Build history of the part. All positions in model axes, mm. Give positions to 0.01 mm unless a question says otherwise; leave off trailing zeros. Write each loop counter-clockwise with the first axis right and the second up, starting at its lowest first coordinate (ties: lowest second). Pieces come first, ordered by that corner, then holes. Notation, with made-up numbers: (-5.75, 49) -> (6.25, 49) arc R22 ccw to (6.25, 88) -> close; hole circle Ø3 at (16, 14). An arc over 180 degrees is marked (long way). One line per question, with ' | ' between items. Start each with the question number.
(1) Band-saw the part on A-A, the plane x = 168.5. Give the cut face in (y, z), and give its area (3 significant figures).
(2) Drill centre lines: probe 1 along X at (y, z) = (162, 5) (3 decimals); probe 2 along Y at (x, z) = (19.05, 2.5); probe 3 along Y at (x, z) = (69, 5.75). Where is each one in solid material? Low to high. Write a range as from..to.
(3) Pin check, flat tips, straight feed: P1, Ø7.5, axis at x = 19.05, y = 127, coming from the +Z side; P2, Ø3, axis at x = 65.5, z = 3, coming from the -Y side; P3, Ø2, axis at y = 90, z = 2, coming from the -X side. Stop position of each tip, or through.
(4) Band-saw the part on C-C, the plane x = 49. Give the cut face in (y, z), and give its area (3 significant figures).
(5) Band-saw the part on B-B, the plane z = 2.5. Count the separate pieces of the cut face and the enclosed holes in it, and give its area (3 significant figures).
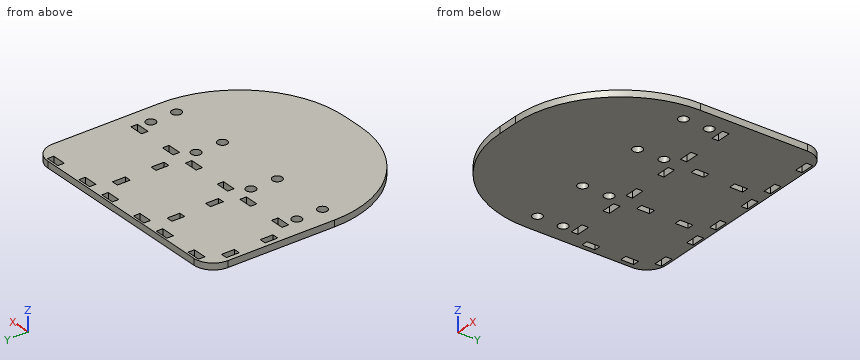
from build123d import *

# Parameters (mm, degrees)
SKETCH1_W               = 228.6
SKETCH1_H               = 228.6
BOSS_EXTRUDE1_DEPTH     = 6.35
CUT_EXTRUDE1_DEPTH      = 324.351577234
CUT_EXTRUDE1_DEPTH_BACK = 324.351577234
SKETCH2_W               = 13.749999996
SKETCH2_H               = 6.35
SKETCH2_W_2             = 13.749999995
CUT_EXTRUDE2_DEPTH      = 324.351577234
CUT_EXTRUDE2_DEPTH_BACK = 324.351577234
SKETCH3_R               = 4.7625
FILLET1_R               = 19.05
FILLET2_R               = 104.14
CUT_EXTRUDE3_DEPTH      = 324.351577234
CUT_EXTRUDE3_DEPTH_BACK = 324.351577234
SKETCH4_W               = 6.35
SKETCH4_H               = 12.7
CUT_EXTRUDE4_DEPTH      = 324.351577234
CUT_EXTRUDE4_DEPTH_BACK = 324.351577234
SKETCH5_R               = 4.7625


with BuildPart() as part:
    # Sketch1 → Boss-Extrude1 (new body)
    with BuildSketch(Plane.XY):
        with Locations((114.3, 114.3)):
            Rectangle(SKETCH1_W, SKETCH1_H)
    extrude(amount=BOSS_EXTRUDE1_DEPTH)

    # Sketch2 → Cut-Extrude1 (cut, two sides: drawn at the far end of the back side and taken through both)
    with BuildSketch(Plane.XY.offset(6.35).offset(-CUT_EXTRUDE1_DEPTH_BACK)):
        with Locations((134.924999993, 223.424999936)):
            Rectangle(SKETCH2_W, SKETCH2_H)
        with Locations((93.675000006, 223.424999936)):
            Rectangle(SKETCH2_W_2, SKETCH2_H)
        with Locations((206.044999993, 223.424999936)):
            Rectangle(SKETCH2_W, SKETCH2_H)
        with Locations((164.795000007, 223.424999936)):
            Rectangle(SKETCH2_W_2, SKETCH2_H)
        with Locations((22.555000007, 223.424999936)):
            Rectangle(SKETCH2_W_2, SKETCH2_H)
        with Locations((63.804999993, 223.424999936)):
            Rectangle(SKETCH2_W, SKETCH2_H)
        with Locations((206.044999993, 140.874999936)):
            Rectangle(SKETCH2_W, SKETCH2_H)
        with Locations((164.795000007, 140.874999936)):
            Rectangle(SKETCH2_W_2, SKETCH2_H)
        with Locations((134.924999993, 140.874999936)):
            Rectangle(SKETCH2_W, SKETCH2_H)
        with Locations((93.675000006, 140.874999936)):
            Rectangle(SKETCH2_W_2, SKETCH2_H)
        with Locations((63.804999993, 140.874999936)):
            Rectangle(SKETCH2_W, SKETCH2_H)
        with Locations((22.555000007, 140.874999936)):
            Rectangle(SKETCH2_W, SKETCH2_H)
    extrude(amount=CUT_EXTRUDE1_DEPTH + CUT_EXTRUDE1_DEPTH_BACK, mode=Mode.SUBTRACT)

    # Sketch3 → Cut-Extrude2 (cut, two sides: drawn at the far end of the back side and taken through both)
    with BuildSketch(Plane.XY.offset(6.35).offset(-CUT_EXTRUDE2_DEPTH_BACK)):
        with Locations((19.05, 127)):
            Circle(SKETCH3_R)
        with Locations(Location((19.05, 101.6, 0), (0, 0, 180))):
            Circle(SKETCH3_R)
        with Locations((209.55, 101.6)):
            Circle(SKETCH3_R)
        with Locations(Location((209.55, 127, 0), (0, 0, 180))):
            Circle(SKETCH3_R)
    extrude(amount=CUT_EXTRUDE2_DEPTH + CUT_EXTRUDE2_DEPTH_BACK, mode=Mode.SUBTRACT)

    # Fillet1
    fillet1_edges = [part.edges().sort_by_distance(p)[0] for p in [
        (0, 228.6, 3.175),
        (228.6, 228.6, 3.175),
    ]]
    fillet(fillet1_edges, radius=FILLET1_R)

    # Fillet2
    fillet2_edges = [part.edges().sort_by_distance(p)[0] for p in [
        (228.6, 0, 3.175),
        (0, 0, 3.175),
    ]]
    fillet(fillet2_edges, radius=FILLET2_R)

    # Sketch4 → Cut-Extrude3 (cut, two sides: drawn at the far end of the back side and taken through both)
    with BuildSketch(Plane.XY.offset(6.35).offset(-CUT_EXTRUDE3_DEPTH_BACK)):
        with Locations((78.74, 201.199999936)):
            Rectangle(SKETCH4_W, SKETCH4_H)
        with Locations((78.74, 163.099999936)):
            Rectangle(SKETCH4_W, SKETCH4_H)
        with Locations((149.86, 163.099999936)):
            Rectangle(SKETCH4_W, SKETCH4_H)
        with Locations((149.86, 201.199999936)):
            Rectangle(SKETCH4_W, SKETCH4_H)
        with Locations((7.62, 163.099999936)):
            Rectangle(SKETCH4_W, SKETCH4_H)
        with Locations((7.62, 201.199999936)):
            Rectangle(SKETCH4_W, SKETCH4_H)
    extrude(amount=CUT_EXTRUDE3_DEPTH + CUT_EXTRUDE3_DEPTH_BACK, mode=Mode.SUBTRACT)

    # Sketch5 → Cut-Extrude4 (cut, two sides: drawn at the far end of the back side and taken through both)
    with BuildSketch(Plane.XY.offset(6.35).offset(-CUT_EXTRUDE4_DEPTH_BACK)):
        with Locations((78.497711148, 127.330967461)):
            Circle(SKETCH5_R)
        with Locations(Location((150.102288852, 127.330967461, 0), (0, 0, 180))):
            Circle(SKETCH5_R)
        with Locations((150.102288852, 101.269032539)):
            Circle(SKETCH5_R)
        with Locations(Location((78.497711148, 101.269032539, 0), (0, 0, 180))):
            Circle(SKETCH5_R)
    extrude(amount=CUT_EXTRUDE4_DEPTH + CUT_EXTRUDE4_DEPTH_BACK, mode=Mode.SUBTRACT)


solid = part.part
Results:
1) outline: (9.77, 0) -> (137.7, 0) -> (137.7, 6.35) -> (9.77, 6.35) -> close; (144.05, 0) -> (220.25, 0) -> (220.25, 6.35) -> (144.05, 6.35) -> close; (226.6, 0) -> (228.6, 0) -> (228.6, 6.35) -> (226.6, 6.35) -> close | area: 1,310 mm²
2) probe 1: x = 0..4.445, 10.795..75.565, 81.915..146.685, 153.035..228.6 | probe 2: y = 44.1..96.84, 106.36..122.24, 131.76..137.7, 144.05..220.25, 226.6..228.6 | probe 3: y = 6.11..137.7, 144.05..220.25, 226.6..228.6
3) P1: passes through | P2: stops at y = 6.85 | P3: stops at x = 0.83
4) outline: (15.8, 0) -> (228.6, 0) -> (228.6, 6.35) -> (15.8, 6.35) -> close | area: 1,350 mm²
5) separate pieces: 1 | enclosed holes: 26 | area: 45,300 mm²
